The listing builds one solid part. Answer for the finished solid, in the listing's coordinates (mm). Give positions to 0.01 mm unless a question says otherwise; leave off trailing zeros. Order: outer loops, then holes, each group sorted by start corner. A loop starts at its lowest first (then second) coordinate and runs counter-clockwise, first axis right, second up.
```python
from build123d import *

# Parameters (mm, degrees)
SKETCH1_R           = 17.5
BOSS_EXTRUDE1_DEPTH = 120
CUT_EXTRUDE1_START  = 30
CUT_EXTRUDE1_DEPTH  = 20
CUT_EXTRUDE2_START  = 90
CUT_EXTRUDE2_DEPTH  = 30
SKETCH3_W           = 1.6
SKETCH3_H           = 1


with BuildPart() as part:
    # Sketch1 → Boss-Extrude1 (new body)
    with BuildSketch(Plane.XY):
        Circle(SKETCH1_R)
    extrude(amount=BOSS_EXTRUDE1_DEPTH)

    # Sketch2 → Cut-Extrude1 (cut)
    with BuildSketch(Plane.XY.offset(CUT_EXTRUDE1_START)):
        with BuildLine():
            Line((-5, 16.770509831), (-5, 12.5))
            Line((-5, 12.5), (5, 12.5))
            Line((5, 12.5), (5, 16.770509831))
            ThreePointArc((5, 16.770509831), (0, 17.5), (-5, 16.770509831))
        make_face()
    extrude(amount=CUT_EXTRUDE1_DEPTH, mode=Mode.SUBTRACT)

    # Sketch2_2 → Cut-Extrude2 (cut)
    with BuildSketch(Plane.XY.offset(CUT_EXTRUDE2_START)):
        with BuildLine():
            Line((-5, 16.770509831), (-5, 12.5))
            Line((-5, 12.5), (5, 12.5))
            Line((5, 12.5), (5, 16.770509831))
            ThreePointArc((5, 16.770509831), (0, 17.5), (-5, 16.770509831))
        make_face()
    extrude(amount=CUT_EXTRUDE2_DEPTH, mode=Mode.SUBTRACT)

    # Sketch3 → Cut-Revolve2 (revolve, cut)
    with BuildSketch(Plane(origin=(0, 0, 0), x_dir=(0, 0, -1), z_dir=(1, 0, 0)), mode=Mode.PRIVATE) as cut_revolve2_sk:
        with Locations((-29.2, 17)):
            Rectangle(SKETCH3_W, SKETCH3_H)
        with Locations((-50.8, 17)):
            Rectangle(SKETCH3_W, SKETCH3_H)
        with Locations((-89.2, 17)):
            Rectangle(SKETCH3_W, SKETCH3_H)
    revolve(cut_revolve2_sk.sketch.rotate(Axis((0, 0, 0), (0, 0, 1)), 90), axis=Axis((0, 0, 0), (0, 0, 1)), mode=Mode.SUBTRACT)


solid = part.part
```
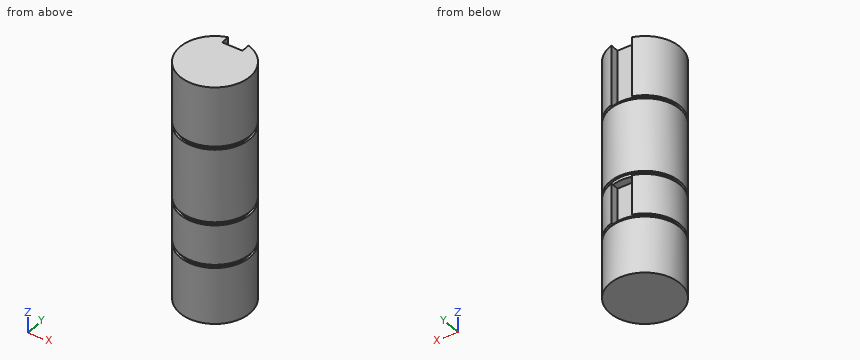
1) Find section B-B (y = 6). Write down the section's boundary in (x, z).
Geometry says:
outline: (-16.44, 0) - (16.44, 0) - (16.44, 28.4) - (15.37, 28.4) - (15.37, 30) - (16.44, 30) - (16.44, 50) - (15.37, 50) - (15.37, 51.6) - (16.44, 51.6) - (16.44, 88.4) - (15.37, 88.4) - (15.37, 90) - (16.44, 90) - (16.44, 120) - (-16.44, 120) - (-16.44, 90) - (-15.37, 90) - (-15.37, 88.4) - (-16.44, 88.4) - (-16.44, 51.6) - (-15.37, 51.6) - (-15.37, 50) - (-16.44, 50) - (-16.44, 30) - (-15.37, 30) - (-15.37, 28.4) - (-16.44, 28.4) - close
2) Given P1, Ø4.5, axis at y = 15, z = 98, coming from the +X side; P2, Ø8, axis at x = 2, z = 42, coming from the +Y side; P3, Ø1.2, axis at x = 2.5, y = 15, coming from the +Z side, each flat-ended and moving along its own axis, determine where each tip first touches the part or whether it passes through.
Geometry says:
P1: stops at x = 11.99
P2: stops at y = 16.77
P3: stops at z = 90
3) Find section A-A (x = 0). Write down the section's boundary in (y, z).
Geometry says:
outline: (-17.5, 0) - (17.5, 0) - (17.5, 28.4) - (16.5, 28.4) - (16.5, 30) - (12.5, 30) - (12.5, 50) - (16.5, 50) - (16.5, 51.6) - (17.5, 51.6) - (17.5, 88.4) - (16.5, 88.4) - (16.5, 90) - (12.5, 90) - (12.5, 120) - (-17.5, 120) - (-17.5, 90) - (-16.5, 90) - (-16.5, 88.4) - (-17.5, 88.4) - (-17.5, 51.6) - (-16.5, 51.6) - (-16.5, 50) - (-17.5, 50) - (-17.5, 30) - (-16.5, 30) - (-16.5, 28.4) - (-17.5, 28.4) - close
4) Straight lines are drawn through the part: probe 1 along Z at (x, y) = (16.5, -3.5); probe 2 along X at (y, z) = (16, 43.5); probe 3 along Y at (x, z) = (-10.5, 14). For each, find the intervals that lie inside material, in ascending order.
Geometry says:
probe 1: z = 0 to 28.4, 30 to 50, 51.6 to 88.4, 90 to 120
probe 2: x = -7.09 to -5, 5 to 7.09
probe 3: y = -14 to 14
5) Find section C-C (z = 10.5). Write down the section's boundary in (x, y), then the cut area to 3 significant figures.
Geometry says:
outline: circle Ø35 at (0, 0)
area: 962 mm2
